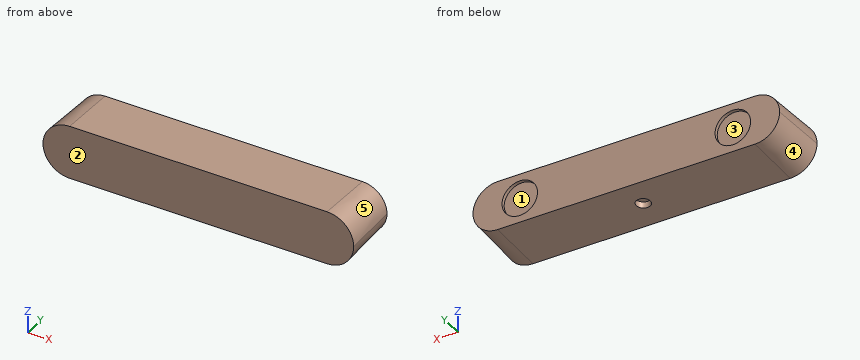
from build123d import *

# Parameters (mm, degrees)
SKETCH1_W           = 175
SKETCH1_H           = 30
BOSS_EXTRUDE1_DEPTH = 33
SKETCH3_R           = 10
CUT_EXTRUDE1_DEPTH  = 2
FILLET1_R           = 15
SKETCH4_R           = 4
CUT_EXTRUDE2_DEPTH  = 4
DRAFT3_ANGLE        = -2


with BuildPart() as part:
    # Sketch1 → Boss-Extrude1 (new body)
    with BuildSketch(Plane(origin=(0, 0, 0), x_dir=(1, 0, 0), z_dir=(0, 1, 0))):
        Rectangle(SKETCH1_W, SKETCH1_H)
    extrude(amount=BOSS_EXTRUDE1_DEPTH)

    # Sketch3 → Cut-Extrude1 (cut)
    with BuildSketch(Plane(origin=(0, 33, 0), x_dir=(1, 0, 0), z_dir=(0, 1, 0))):
        with Locations(Location((-60, 0, 0), (0, 0, 270))):
            Circle(SKETCH3_R)
        with Locations(Location((60, 0, 0), (0, 0, 270))):
            Circle(SKETCH3_R)
    extrude(amount=-CUT_EXTRUDE1_DEPTH, mode=Mode.SUBTRACT)

    # Fillet1
    fillet1_edges = [part.edges().sort_by_distance(p)[0] for p in [
        (-87.5, 16.5, -15),
        (87.5, 16.5, 15),
        (87.5, 16.5, -15),
        (-87.5, 16.5, 15),
    ]]
    fillet(fillet1_edges, radius=FILLET1_R - 0.0001)  # a hair under: the kernel refuses the full size

    # Sketch4 → Cut-Extrude2 (cut)
    with BuildSketch(Plane(origin=(0, 0, -15), x_dir=(-1, 0, 0), z_dir=(0, 0, -1))):
        with Locations((0, 17.1)):
            Circle(SKETCH4_R)
    extrude(amount=-CUT_EXTRUDE2_DEPTH, mode=Mode.SUBTRACT)

    # Draft3
    draft3_faces = [part.faces().sort_by_distance(p)[0] for p in [
        (0, 16.5, 15),
        (83.106631007, 16.5, 10.606631007),
        (83.106631007, 16.5, -10.606631007),
        (0, 1.487079621, -15),
        (-83.106631007, 16.5, 10.606631007),
        (-83.106631007, 16.5, -10.606631007),
    ]]
    draft(draft3_faces, Plane(origin=(0, 0, 0), x_dir=(0, 0, -1), z_dir=(0, -1, 0)), DRAFT3_ANGLE)


solid = part.part
Can you work these out from the model? Positions are in its coordinate system, mm. Face numbers are marked on the shaded views. A direction names the side the tool comes from. Coordinates: 2 decimals unless noted, no trailing zeros. Write each loop counter-clockwise with the first axis right and the second up, starting at its lowest first coordinate (ties: lowest second). Pieces come first, ordered by that corner, then holes.
Q1. Imagine slicing it at D-D, the plane x = -6. List the corners of the cut face in (y, z) for me, plus the area to 3 significant figures.
Results found:
outline: (0, -15) - (33, -13.85) - (33, 13.85) - (0, 15) - close
area: 952 mm2
Q2. Please list where these lines run through material, in increasing order: L1, parallel to X at y = 32.45, z = 0; L2, parallel to Y at x = 0, z = -13.4; L3, parallel to Z at x = 57.5, y = 31.5.
Results found:
L1: x = -86.37 to -70, -50 to 50, 70 to 86.37
L2: y = 0 to 13.1, 21.1 to 33
L3: z = -13.9 to -9.68, 9.68 to 13.9
Q3. Imagine slicing it at A-A, the plane x = 60. List the corners of the cut face in (y, z) for me.
Results found:
outline: (0, -15) - (33, -13.85) - (33, -10) - (31, -10) - (31, 10) - (33, 10) - (33, 13.85) - (0, 15) - close
Q4. If we mould it in two halves opening along X, with no side actions, what happens to the marked faces 3, 4 and 5? For each: +X half, -X half, draft (parallel to the pull), parting line (faces both ways), or undercut.
Results found:
face 3: undercut
face 4: -X half
face 5: +X half
Q5. For P1, Ø1.5, axis at x = -52.5, z = -5, coming from the +Y side; P2, Ø6.5, axis at x = -1.5, y = 15.5, coming from the -Z side; P3, Ø6.5, axis at x = 0, y = 17.1, coming from the -Z side, each with a flat end and sliding along its axis, tell me the tip position at first contact or that it passes through.
Results found:
P1: stops at y = 31
P2: stops at z = -14.57
P3: stops at z = -11
Q6. Which directions (+Z, -Z, +X, -X, +Y, -Y) give clear straight access to the entire face, cutting with the end or side of a thin tool? Please do the marked faces 1 and 2.
Results found:
face 1: +Y
face 2: +Z, -Z, +X, -X, -Y
